Source: three-view drawing plus pictorial views. Frame: mm from the lowest corner of the part. A direction names the side the tool comes from. Round coordinates to 2 decimals unless told otherwise and drop trailing zeros. Write each loop counter-clockwise with the first axis right and the second up, starting at its lowest first coordinate (ties: lowest second). Pieces come first, ordered by that corner, then holes. Notation, with made-up numbers: (76.5, -39.75) -> (89.5, -39.75) arc R14 ccw to (89.5, -28.75) -> close; hole circle Ø10 at (12.25, -10.75). An arc over 180 degrees is marked (long way). Put each result on its own line as item: value.
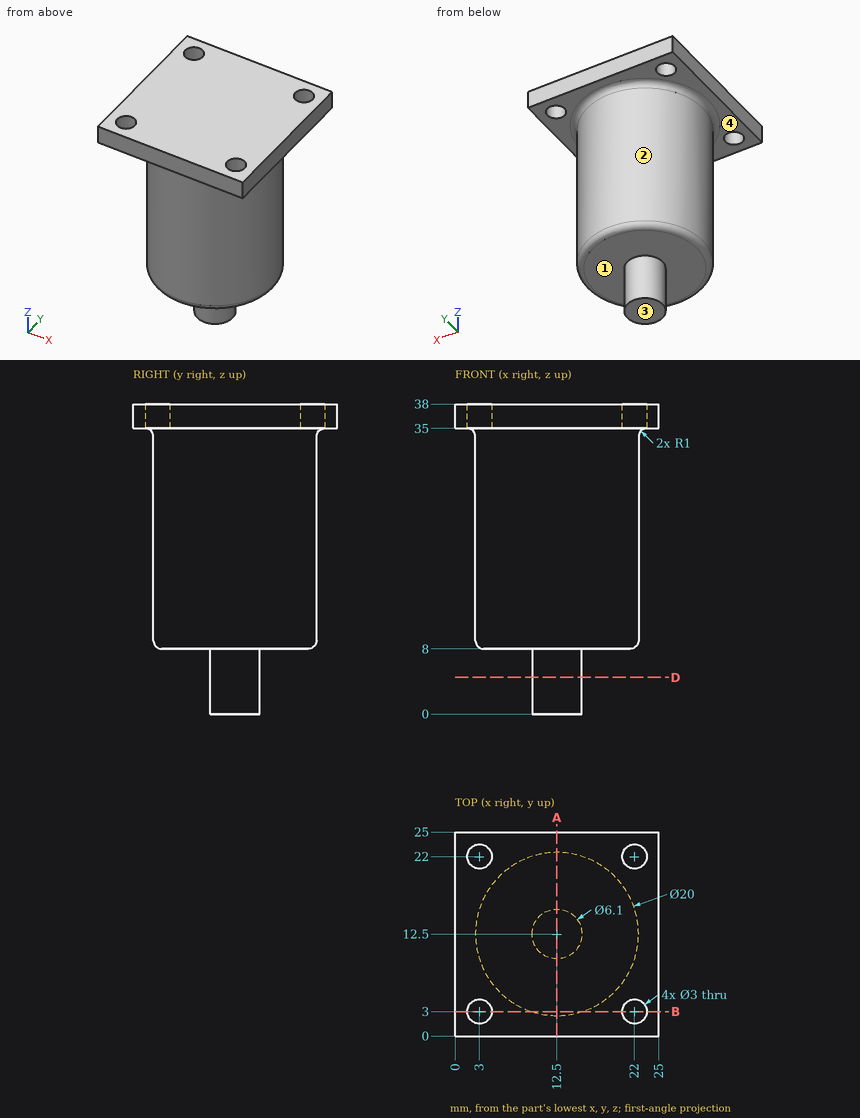
Q1. Pin query (flat end, axial travel): pin 1 (6 mm diameter, centred on y = 11.5, z = 22.5, fed in from +X); pin 2 (2 mm diameter, centred on x = 18, z = 24, fed in from +Y); pin 3 (2 mm diameter, centred on y = 18.5, z = 23.5, fed in from +X). Return the tip coordinate at first contact, or that it passes through.
Ans:
pin 1: stops at x = 22.5
pin 2: stops at y = 21.43
pin 3: stops at x = 21.16
Q2. Cut plane B-B on y = 3. Give the number of separate pieces and of enclosed holes in the cut face, and give its area (3 significant figures).
Ans:
separate pieces: 3
enclosed holes: 0
area: 225 mm^2
Q3. Material intervals for line 1 (Y direction, x = 3, z = 36.7); line 2 (Z direction, x = 23.25, y = 6); line 3 (Z direction, x = 5.25, y = 10.5), sorted ascending. Write a range as [from, to].
Ans:
line 1: y = [0, 1.5], [4.5, 20.5], [23.5, 25]
line 2: z = [35, 38]
line 3: z = [8, 38]
Q4. Cut plane A-A on x = 12.5. Output: boundary loops of the cut face in (y, z), and give its area (3 significant figures).
Ans:
outline: (0, 35) -> (1.5, 35) arc R1 cw to (2.5, 34) -> (2.5, 9) arc R1 ccw to (3.5, 8) -> (9.45, 8) -> (9.45, 0) -> (15.55, 0) -> (15.55, 8) -> (21.5, 8) arc R1 ccw to (22.5, 9) -> (22.5, 34) arc R1 cw to (23.5, 35) -> (25, 35) -> (25, 38) -> (0, 38) -> close
area: 664 mm^2
Q5. Draft query along Y for the marked faces 1 and 2. Return one class per face: +Y half, -Y half, draft (parallel to the pull), parting line (faces both ways), or undercut.
Ans:
face 1: draft
face 2: parting line
Q6. Cut plane D-D on z = 4.5. Output: boundary loops of the cut face in (x, y), and give its area (3 significant figures).
Ans:
outline: circle Ø6.1 at (12.5, 12.5)
area: 29.2 mm^2
Q7. Reachability of the marked faces 3 and 4 from +Z, -Z, +X, -X, +Y, -Y: full face, straight path, thin tool, end or side. Return the list, or none.
Ans:
face 3: -Z, +X, -X, +Y, -Y
face 4: -Z
